For this review, take the finished solid that the model builds, in its own axes (mm). Face numbers are marked on the shaded views. Coordinates: 2 decimals unless noted, no trailing zeros. Order: outer loops, then holes, each group sorted by start corner. A loop starts at its lowest first (then second) coordinate and runs counter-clockwise, first axis right, second up.
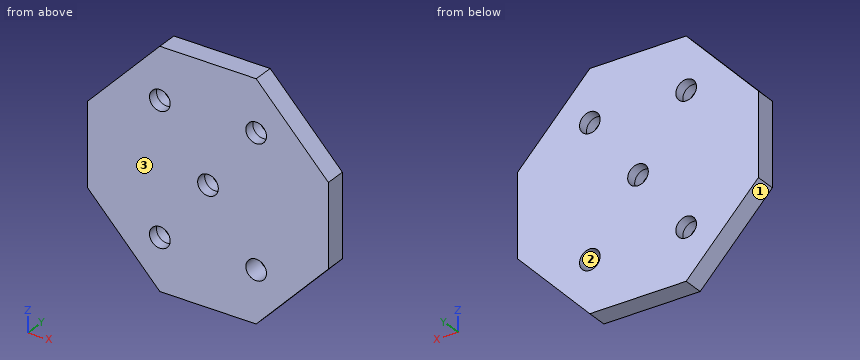
from build123d import *

# Parameters (mm, degrees)
SKETCH1_R           = 1.5
BOSS_EXTRUDE1_DEPTH = 1.5


with BuildPart() as part:
    # Sketch1 → Boss-Extrude1 (new body, symmetric)
    with BuildSketch(Plane(origin=(0, 0, 0), x_dir=(1, 0, 0), z_dir=(0, 1, 0))):
        with BuildLine():
            Line((1.5, 0), (17.5, 0))
            Line((17.5, 0), (17.5, 6))
            Line((17.5, 6), (7, 17))
            Line((7, 17), (0, 17))
            Line((0, 17), (-7, 17))
            Line((-7, 17), (-17.5, 6))
            Line((-17.5, 6), (-17.5, 0))
            Line((-17.5, 0), (-1.5, 0))
            ThreePointArc((-1.5, 0), (0, 1.5), (1.5, 0))
        make_face()
        with Locations((-7, 9.5)):
            Circle(SKETCH1_R, mode=Mode.SUBTRACT)
        with Locations((7, 9.5)):
            Circle(SKETCH1_R, mode=Mode.SUBTRACT)
        with BuildLine():
            Line((7, -17), (17.5, -6))
            Line((17.5, -6), (17.5, 0))
            Line((17.5, 0), (1.5, 0))
            ThreePointArc((1.5, 0), (0, -1.5), (-1.5, 0))
            Line((-1.5, 0), (-17.5, 0))
            Line((-17.5, 0), (-17.5, -6))
            Line((-17.5, -6), (-7, -17))
            Line((-7, -17), (0, -17))
            Line((0, -17), (7, -17))
        make_face()
        with Locations((-7, -9.5)):
            Circle(SKETCH1_R, mode=Mode.SUBTRACT)
        with Locations((7, -9.5)):
            Circle(SKETCH1_R, mode=Mode.SUBTRACT)
    extrude(amount=BOSS_EXTRUDE1_DEPTH, both=True)


solid = part.part
1. Clearance check with flat-ended pins moving along their axes: pin 1 Ø1 at (y, z) = (-1, -9.5) entering from -X; pin 2 Ø2.5 at (x, z) = (7, 9.5) entering from +Y; pin 3 Ø1.5 at (x, y) = (13, -0.5) entering from +Z. State where each tip first meets the part, or that it passes through.
Answer below:
pin 1: stops at x = -14.64
pin 2: passes through
pin 3: stops at z = 11.5
2. Take a section at A-A, the plane y = -1. Give the boundary of the cut face in (x, z).
Answer below:
outline: (-17.5, -6) - (-7, -17) - (7, -17) - (17.5, -6) - (17.5, 6) - (7, 17) - (-7, 17) - (-17.5, 6) - close; hole circle Ø3 at (-7, -9.5); hole circle Ø3 at (-7, 9.5); hole circle Ø3 at (0, 0); hole circle Ø3 at (7, -9.5); hole circle Ø3 at (7, 9.5)
3. To check wall thickness, follow L1, parallel to Z at x = 7, y = -0.8; L2, parallel to Z at x = 8, y = 0.6; L3, parallel to X at y = -0.8, z = -9.5. State the ranges of each line that lie inside material, in increasing order.
Answer below:
L1: z = -17 to -11, -8 to 8, 11 to 17
L2: z = -15.95 to -10.62, -8.38 to 8.38, 10.62 to 15.95
L3: x = -14.16 to -8.5, -5.5 to 5.5, 8.5 to 14.16
4. The part is to be moulded in two halves that separate along Z. For the marked faces 1, 2 and 3, say which applies: +Z half, -Z half, draft (parallel to the pull), parting line (faces both ways), or undercut.
Answer below:
face 1: -Z half
face 2: undercut
face 3: draft
5. Take a section at C-C, the plane z = 0. Give the boundary of the cut face in (x, y), plus the area to 3 significant figures.
Answer below:
outline: (-17.5, -1.5) - (-1.5, -1.5) - (-1.5, 1.5) - (-17.5, 1.5) - close; (1.5, -1.5) - (17.5, -1.5) - (17.5, 1.5) - (1.5, 1.5) - close
area: 96.0 mm2
6. Take a section at D-D, the plane z = 9.5. Give the boundary of the cut face in (x, y), plus the area to 3 significant figures.
Answer below:
outline: (-14.16, -1.5) - (-8.5, -1.5) - (-8.5, 1.5) - (-14.16, 1.5) - close; (-5.5, -1.5) - (5.5, -1.5) - (5.5, 1.5) - (-5.5, 1.5) - close; (8.5, -1.5) - (14.16, -1.5) - (14.16, 1.5) - (8.5, 1.5) - close
area: 67.0 mm2
7. Take a section at B-B, the plane x = 0. Give the boundary of the cut face in (y, z), plus the area to 3 significant figures.
Answer below:
outline: (-1.5, -17) - (1.5, -17) - (1.5, -1.5) - (-1.5, -1.5) - close; (-1.5, 1.5) - (1.5, 1.5) - (1.5, 17) - (-1.5, 17) - close
area: 93.0 mm2
